Could you check a few things on this model? Use its own coordinates, in mm. Face numbers are marked on the shaded views. A direction names the side the tool comes from. Give positions to 0.01 mm unless a question says otherwise; leave off trailing zeros. Order: outer loops, then holes, each group sorted by start corner. A loop starts at its lowest first (then second) coordinate and runs counter-clockwise, first axis right, second up.
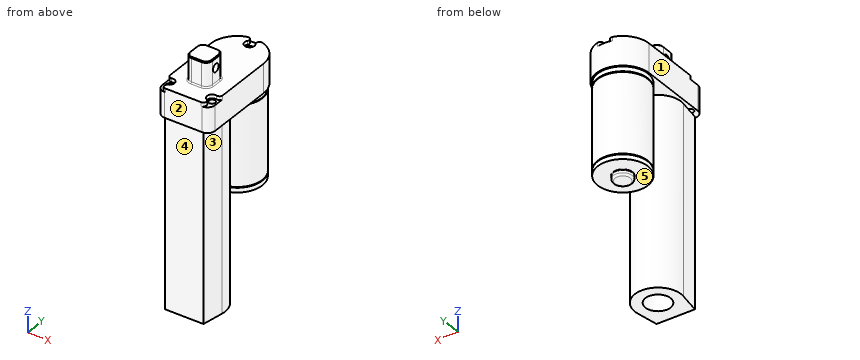
from build123d import *

# Parameters (mm, degrees)
BOSS_EXTRUDE1_DEPTH            = 23
CUT_EXTRUDE1_DEPTH             = 3
CUT_EXTRUDE2_DEPTH             = 3
CUT_EXTRUDE3_DEPTH             = 3
SKETCH5_W                      = 18
SKETCH5_H                      = 18
BOSS_EXTRUDE2_DEPTH            = 20
BOSS_EXTRUDE3_DEPTH            = 149.7
SKETCH8_W                      = 10
SKETCH8_H                      = 138
F_5_0_5_DIAMETER_HOLE1_D       = 5
F_5_0_5_DIAMETER_HOLE1_DEPTH   = 20
F_6_4_6_4_DIAMETER_HOLE1_D     = 6.4
F_6_4_6_4_DIAMETER_HOLE1_DEPTH = 30
FILLET1_R                      = 5
CHAMFER1_SIZE                  = 0.657
FILLET2_R                      = 0.5
FILLET3_R                      = 1
FILLET4_R                      = 1.5
FILLET5_START                  = -35.454500108
FILLET5_DEPTH                  = 4.454500108
FILLET6_R                      = 6
SKETCH19_R                     = 10
CUT_EXTRUDE4_DEPTH             = 30
SCALE1_SCALE                   = 0.5


with BuildPart() as part:
    # Sketch1 → Boss-Extrude1 (new body)
    with BuildSketch(Plane.XY.offset(-32.454500108)):
        with BuildLine():
            Line((13.42953052, -65.776710579), (55.42953052, -65.776710579))
            Line((55.42953052, -65.776710579), (55.42953052, -4.776710579))
            ThreePointArc((55.42953052, -4.776710579), (34.42953052, 16.223289421), (13.42953052, -4.776710579))
            Line((13.42953052, -4.776710579), (13.42953052, -65.776710579))
        make_face()
    extrude(amount=-BOSS_EXTRUDE1_DEPTH)

    # Sketch2 → Cut-Extrude1 (cut)
    with BuildSketch(Plane.XY.offset(-32.454500108)):
        with BuildLine():
            Line((13.42953052, -57.351010373), (13.42953052, -65.776710579))
            Line((13.42953052, -65.776710579), (20.100874204, -65.776710579))
            ThreePointArc((20.100874204, -65.776710579), (17.656719067, -63.802168161), (19.073434325, -60.997595115))
            ThreePointArc((19.073434325, -60.997595115), (19.600289003, -53.991277109), (13.42953052, -57.351010373))
        make_face()
    extrude(amount=-CUT_EXTRUDE1_DEPTH, mode=Mode.SUBTRACT)

    # Sketch3 → Cut-Extrude2 (cut)
    with BuildSketch(Plane.XY.offset(-32.454500108)):
        with BuildLine():
            Line((55.42953052, -65.776710579), (55.42953052, -57.394966506))
            ThreePointArc((55.42953052, -57.394966506), (49.285998633, -54.017797418), (49.726894996, -61.01450132))
            ThreePointArc((49.726894996, -61.01450132), (51.102575978, -63.821906348), (48.662747793, -65.776710579))
            Line((48.662747793, -65.776710579), (55.42953052, -65.776710579))
        make_face()
    extrude(amount=-CUT_EXTRUDE2_DEPTH, mode=Mode.SUBTRACT)

    # Sketch4 → Cut-Extrude3 (cut)
    with BuildSketch(Plane.XY.offset(-32.454500108)):
        with BuildLine():
            ThreePointArc((28.400368742, 15.33918384), (31.143729281, 14.409675692), (31.167916073, 11.513224857))
            ThreePointArc((31.167916073, 11.513224857), (34.442423035, 5.223292745), (37.733137686, 11.504760638))
            ThreePointArc((37.733137686, 11.504760638), (37.764792889, 14.401139479), (40.510541043, 15.323570788))
            ThreePointArc((40.510541043, 15.323570788), (34.456604769, 16.223271968), (28.400368742, 15.33918384))
        make_face()
    extrude(amount=-CUT_EXTRUDE3_DEPTH, mode=Mode.SUBTRACT)

    # Sketch5 → Boss-Extrude2 (add)
    with BuildSketch(Plane.XY.offset(-32.454500108)):
        with Locations((34.42953052, -41.776710579)):
            Rectangle(SKETCH5_W, SKETCH5_H)
    extrude(amount=BOSS_EXTRUDE2_DEPTH)

    # Sketch6 → Boss-Extrude3 (add)
    with BuildSketch(Plane(origin=(0, 0, -55.454500108), x_dir=(-1, 0, 0), z_dir=(0, 0, -1))):
        with BuildLine():
            Line((-16.172658971, -47.421015636), (-19.022097723, -64.486635224))
            Line((-19.022097723, -64.486635224), (-49.522097723, -64.486635224))
            Line((-49.522097723, -64.486635224), (-52.371536476, -47.421015636))
            ThreePointArc((-52.371536476, -47.421015636), (-34.272097723, -26.048960567), (-16.172658971, -47.421015636))
        make_face()
    extrude(amount=BOSS_EXTRUDE3_DEPTH)

    # Sketch7 → Revolve1 (revolve)
    with BuildSketch(Plane.XZ.offset(4.776710579), mode=Mode.PRIVATE) as revolve1_sk:
        Polygon((54.42953052, -55.454500108), (34.42953052, -55.454500108), (34.42953052, -131.454500108), (41.92953052, -131.454500108), (41.92953052, -127.454500108), (54.42953052, -127.454500108), (54.42953052, -123.754500108), (54.12953052, -123.454500108), (54.42953052, -123.154500108), (54.42953052, -59.754500108), (54.12953052, -59.454500108), (54.42953052, -59.154500108), align=None)
    revolve(revolve1_sk.sketch.rotate(Axis((34.42953052, -4.776710579, -55.454500108), (0, 0, -1)), 180), axis=Axis((34.42953052, -4.776710579, -55.454500108), (0, 0, -1)))

    # Sketch8 → Cut-Revolve1 (revolve, cut)
    with BuildSketch(Plane(origin=(0, -44.398960567, 0), x_dir=(1, 0, 0), z_dir=(0, 1, 0))):
        with Locations((39.272097723, 116.154500108)):
            Rectangle(SKETCH8_W, SKETCH8_H)
    revolve(axis=Axis((34.272097723, -44.398960567, -185.154500108), (0, 0, 1)), mode=Mode.SUBTRACT)

    # Ø5.0 (5) Diameter Hole1
    with Locations(Plane.XY.offset(-35.454500108)):
        with Locations((34.447580034, 9.223289421), (17.42953052, -57.351010373), (51.42953052, -57.394966506)):
            Hole(F_5_0_5_DIAMETER_HOLE1_D / 2, depth=F_5_0_5_DIAMETER_HOLE1_DEPTH)

    # Ø6.4 (6.4) Diameter Hole1
    with Locations(Plane(origin=(43.42953052, 0, 0), x_dir=(0, 0, -1), z_dir=(1, 0, 0))):
        with Locations((20.454500108, -41.749998068)):
            Hole(F_6_4_6_4_DIAMETER_HOLE1_D / 2, depth=F_6_4_6_4_DIAMETER_HOLE1_DEPTH)

    # Fillet1
    fillet1_edges = [part.edges().sort_by_distance(p)[0] for p in [
        (25.42953052, -32.776710579, -22.454500108),
        (25.42953052, -50.776710579, -22.454500108),
        (43.42953052, -50.776710579, -22.454500108),
        (43.42953052, -32.776710579, -22.454500108),
    ]]
    fillet(fillet1_edges, radius=FILLET1_R)

    # Chamfer1
    chamfer1_edges = [part.edges().sort_by_distance(p)[0] for p in [
        (25.42953052, -41.776710579, -12.454500108),
        (34.42953052, -32.776710579, -12.454500108),
        (34.42953052, -50.776710579, -12.454500108),
        (43.42953052, -41.776710579, -12.454500108),
        (41.965064426, -34.241176673, -12.454500108),
        (26.893996615, -49.312244485, -12.454500108),
        (41.965064426, -49.312244485, -12.454500108),
        (26.893996615, -34.241176673, -12.454500108),
    ]]
    chamfer(chamfer1_edges, length=CHAMFER1_SIZE)

    # Fillet2
    fillet2_edges = [part.edges().sort_by_distance(p)[0] for p in [
        (41.92953052, -4.776710579, -127.454500108),
        (24.272097723, -44.398960567, -185.154500108),
    ]]
    fillet(fillet2_edges, radius=FILLET2_R)

    # Fillet3
    fillet3_edges = [part.edges().sort_by_distance(p)[0] for p in [
        (25.42953052, -41.776710579, -32.454500108),
        (34.42953052, -32.776710579, -32.454500108),
        (43.42953052, -41.776710579, -32.454500108),
        (34.42953052, -50.776710579, -32.454500108),
        (26.893996615, -34.241176673, -32.454500108),
        (41.965064426, -49.312244485, -32.454500108),
        (26.893996615, -49.312244485, -32.454500108),
        (41.965064426, -34.241176673, -32.454500108),
    ]]
    fillet(fillet3_edges, radius=FILLET3_R)

    # Fillet4
    fillet4_edges = [part.edges().sort_by_distance(p)[0] for p in [
        (41.92953052, -4.776710579, -131.454500108),
    ]]
    fillet(fillet4_edges, radius=FILLET4_R)

    # Fillet5: read off the stored shape, not the designer's step
    # Fillet5 outline → Fillet5 (cut)
    with BuildSketch(Plane.XY.offset(FILLET5_START)):
        with BuildLine():
            ThreePointArc((16.506453597, -53.45897633), (14.379096338, -52.987616404), (13.42953052, -51.026455053))
            Line((13.42953052, -51.026455053), (13.42953052, -57.351010373))
            ThreePointArc((13.42953052, -57.351010373), (14.291672358, -54.870315681), (16.506453597, -53.45897633))
        make_face()
        with BuildLine():
            ThreePointArc((55.42953052, -51.070411186), (54.479964703, -53.031572537), (52.352607444, -53.502932463))
            ThreePointArc((52.352607444, -53.502932463), (54.567388683, -54.914271815), (55.42953052, -57.394966506))
            Line((55.42953052, -57.394966506), (55.42953052, -51.070411186))
        make_face()
    extrude(amount=FILLET5_DEPTH, mode=Mode.SUBTRACT)

    # Fillet6
    fillet6_edges = [part.edges().sort_by_distance(p)[0] for p in [
        (55.42953052, -65.776710579, -45.454500108),
        (13.42953052, -65.776710579, -45.454500108),
    ]]
    fillet(fillet6_edges, radius=FILLET6_R)

    # Sketch19 → Cut-Extrude4 (cut)
    with BuildSketch(Plane(origin=(0, 0, -205.154500108), x_dir=(-1, 0, 0), z_dir=(0, 0, -1))):
        with Locations(Location((-34.272097723, -44.398960567, 0), (0, 0, 180))):
            Circle(SKETCH19_R)
    extrude(amount=-CUT_EXTRUDE4_DEPTH, mode=Mode.SUBTRACT)


with BuildPart() as part_1:
    # Scale1: scaled about (34.360705618, -29.246210069, -96.472143376)
    add(part.part.scale(SCALE1_SCALE).moved(Location((17.180352809, -14.623105034, -48.236071688))))


solid = part_1.part
Item 1: Imagine slicing it at A-A on z = -95. List the corners of the cut face in (x, y) for me (3 decimals), then the cut area to 3 significant figures.
Findings:
outline: circle Ø20 at (34.395, -17.011); (25.267, -38.334) - (26.691, -46.866) - (41.941, -46.866) - (43.366, -38.334) arc R9.175 ccw (long way) to start; hole circle Ø10 at (34.316, -36.823)
area: 538 mm2
Item 2: Imagine slicing it at B-B on z = -131.5. List the corners of the cut face in (x, y) for me (3 decimals).
Findings:
outline: (25.267, -38.334) - (26.691, -46.866) - (41.941, -46.866) - (43.366, -38.334) arc R9.175 ccw (long way) to start; hole circle Ø10 at (34.316, -36.823)
Item 3: Please list where these lines run through material, in increasing order: line 1 along Y through (x, z) = (34.25, -94.5); line 2 along Y through (x, z) = (37.5, -110); line 3 along Z through (x, y) = (44.25, -35.5).
Findings:
line 1: y = -46.87 to -41.82, -31.82 to -27.65, -27.01 to -7.01
line 2: y = -46.87 to -40.68, -32.97 to -28.22, -26.4 to -7.62
line 3: z = -75.96 to -64.46
Item 4: For pin 1 (12 mm diameter, centred on x = 33.5, y = -20.5, fed in from +Z); pin 2 (9 mm diameter, centred on x = 34.32, y = -36.82, fed in from -Z); pin 3 (4.5 mm diameter, centred on x = 36.5, z = -103, fed in from -Y), each with a flat end and sliding along its axis, tell me the tip position at first contact or that it passes through.
Findings:
pin 1: stops at z = -64.46
pin 2: stops at z = -71.81
pin 3: stops at y = -46.87
Item 5: For the marked faces 1, 2, 3, 4 and 5, which set-ups out of +Z, -Z, +X, -X, +Y, -Y let a thin tool reach every point of the face, with its end or its side?
Findings:
face 1: +Z, -Z, -X, +Y, -Y
face 2: +Z, -Z, +X, -X, -Y
face 3: -Z, +X, -Y
face 4: -Z, +X, -X, -Y
face 5: -Z
